Geometry: final body of the model. Coordinates: model frame, mm. Coordinates: 2 decimals unless noted, no trailing zeros. Loops run counter-clockwise (first coordinate to the right, second up) from the corner with the lowest first, then second, coordinate; pieces in that order, holes last. Notation, with made-up numbers: (81, 4) -> (96, 4) arc R33 ccw to (96, 34) -> close; hole circle Ø5 at (32, 67). An arc over 180 degrees is marked (long way). One line per item, written item: value. Start each with the question number.
Item 1: Mould query, pull axis X, two halves, no side actions, for faces 1 (the cylindrical face through (25.075, 22.373, 7.897)), 2 (the flat face through (0, 23.178, 0)), 3 (the cylindrical face through (-17.733, 21.751, -11.589)). Classes: +X half, -X half, draft (parallel to the pull), parting line (faces both ways), or undercut.
Item 2: Section query D-D on x = -7. Return loops of the section in (y, z).
Item 3: Ray query, probe 1 along Z at (x, y) = (-20, 21.9); probe 2 along X at (y, z) = (23, 10); probe 3 along X at (y, z) = (22.5, 7.5). Return the intervals inside material, ascending. Write a range as from..to.
Item 4: Section query A-A on x = 0. Return loops of the section in (y, z), then the cut area to 3 significant figures.
Item 5: Section query B-B on y = 22.7. Give the number of separate pieces and of enclosed holes in the cut face, then the cut area to 3 significant figures.
Item 6: Contact query for a flat-ended pin moving along its axis: pin 1 Ø5 at (x, z) = (-19.25, -11.11) entering from -Y. Output: stop coordinate, or through.
Item 7: Section query C-C on z = 4. Return loops of the section in (x, y).
Autodesk Inventor part; units mm, degrees
ref_plane "Work Plane1" through (0, 21.59, 0) normal (0, 1, 0) x (1, 0, 0)
ref_plane "YZ Plane" through (0, 0, 0) normal (1, 0, 0) x (0, 1, 0)
ref_plane "XZ Plane" through (0, 0, 0) normal (0, 1, 0) x (-1, 0, 0)
sketch "Sketch6" plane through (0, 0, 0) normal (0, 0, 1) x (1, 0, 0)
  line L0 (540.6478, 1219.1491) -> (540.6478, -58.7076) construction
  line L1 (540.6478, -58.7076) -> (-407.4394, -58.7076) construction
  line L2 (-407.4394, -58.7076) -> (-407.4394, 1219.1491) construction
  line L3 (-407.4394, 1219.1491) -> (540.6478, 1219.1491) construction
  point P0 (0, 0)
sketch "Sketch5" plane through (0, 0, 0) normal (0, 0, 1) x (1, 0, 0)
  line L0 (0, 0) -> (0, 142.24)
  line L1 (0, 142.24) -> (50.8, 142.24)
  line L2 (50.8, 142.24) -> (-50.8, 142.24)
  line L3 (50.8, 142.24) -> (45.2986, 0) construction
  line L4 (45.2986, 0) -> (0, 0) construction
  spline S0 degree 2 poles (50.8, 142.24) (45.2986, 0) (0, 0) knots 1 1 1 2 2 2
  line L5 (-50.8, 142.24) -> (-45.2986, 0) construction
  line L6 (-45.2986, 0) -> (0, 0) construction
  spline S1 degree 2 poles (-50.8, 142.24) (-45.2986, 0) (0, 0) knots 1 1 1 2 2 2
  dimension "d20" = 142.24
  dimension "d21" = 50.8
  dimension "d22" = 101.6
revolve "Revolution1" add sketch "Sketch5" angle 360 about axis through (0, 0, 0) along (0, 1, 0) contours L0 L1 S0
ref_plane "Work Plane1" through (0, 21.59, 0) normal (0, 1, 0) x (1, 0, 0)
sketch "Sketch9" plane through (0, 21.59, 0) normal (0, 1, 0) x (1, 0, 0)
  line L0 (-101.4531, 67.0538) -> (104.6936, 67.0538)
  line L1 (104.6936, 67.0538) -> (104.6936, -70.5436)
  line L2 (104.6936, -70.5436) -> (-101.4531, -70.5436)
  line L3 (-101.4531, -70.5436) -> (-101.4531, 67.0538)
  point P0 (0, 0)
extrude "Extrusion2" cut sketch "Sketch9" along normal through all
sketch "Sketch10" plane through (0, 21.59, 0) normal (0, 1, 0) x (1, 0, 0)
  circle A0 centre (0, 0) radius 29.2557
  circle A1 centre (0, 0) radius 26.289
  dimension "d75" = 58.5114
  dimension "d76" = 52.578
extrude "Extrusion3" add sketch "Sketch10" along normal blind 1.5875 contours A1
extrude "Extrusion4" cut sketch "Sketch10" against normal through all contours A0 | A1
sketch "Sketch11" plane through (0, 23.1775, 0) normal (0, 1, 0) x (1, 0, 0)
  line L0 (0, 0) -> (0, 22.225)
  circle A0 centre (0, 22.225) radius 1.5875
  circle A1 centre (-19.2474, 11.1125) radius 1.5875
  circle A2 centre (-19.2474, -11.1125) radius 1.5875
  circle A3 centre (0, -22.225) radius 1.5875
  circle A4 centre (19.2474, -11.1125) radius 1.5875
  circle A5 centre (19.2474, 11.1125) radius 1.5875
  dimension "d81" = 22.225
  dimension "d82" = 3.175
  dimension "d85" = 360
extrude "Extrusion5" cut sketch "Sketch11" against normal blind 1.5875
chamfer "Chamfer1" distance 1.27 angle 45 6 edges at (17.6599, 23.1775, 11.1125) (17.6599, 23.1775, -11.1125) (-1.5875, 23.1775, -22.225) (-20.8349, 23.1775, -11.1125) (-20.8349, 23.1775, 11.1125) (-1.5875, 23.1775, 22.225)
sketch "Sketch12" plane through (0, 23.1775, 0) normal (0, 1, 0) x (1, 0, 0)
  line L0 (0, 0) -> (11.5101, -5.3673)
  line L1 (0, 0) -> (12.7, 0) construction
  circle A0 centre (11.5101, -5.3673) radius 3.175
  circle A1 centre (-11.5101, -5.3673) radius 3.175
  line L2 (0, 0) -> (-11.5101, -5.3673) construction
  dimension "d92" = 12.7
  dimension "d93" = 25
  dimension "d94" = 6.35
  dimension "d95" = 6.35
extrude "Extrusion6" cut sketch "Sketch12" against normal through all
properties part number "foreHullInsert"
Reply:
1. face 1: parting line
1. face 2: draft
1. face 3: undercut
2. outline: (21.59, -25.34) -> (23.18, -25.34) -> (23.18, 25.34) -> (21.59, 25.34) -> close
3. probe 1: z = -17.06..-12.51, -9.71..9.71, 12.51..17.06
3. probe 2: x = -24.31..-21.69, -16.81..16.81, 21.69..24.31
3. probe 3: x = -25.2..-13.86, -9.16..9.16, 13.86..25.2
4. outline: (21.59, -26.29) -> (23.18, -26.29) -> (23.18, -25.08) -> (21.91, -23.81) -> (21.59, -23.81) -> close; (21.59, -20.64) -> (21.91, -20.64) -> (23.18, -19.37) -> (23.18, 19.37) -> (21.91, 20.64) -> (21.59, 20.64) -> close; (21.59, 23.81) -> (21.91, 23.81) -> (23.18, 25.08) -> (23.18, 26.29) -> (21.59, 26.29) -> close
4. area: 70.2 mm²
5. separate pieces: 1
5. enclosed holes: 8
5. area: 2,000 mm²
6. pin 1: stops at y = 21.59
7. outline: (-25.98, 21.59) -> (-14.38, 21.59) -> (-14.38, 23.18) -> (-25.98, 23.18) -> close; (-8.64, 21.59) -> (8.64, 21.59) -> (8.64, 23.18) -> (-8.64, 23.18) -> close; (14.38, 21.59) -> (25.98, 21.59) -> (25.98, 23.18) -> (14.38, 23.18) -> close
